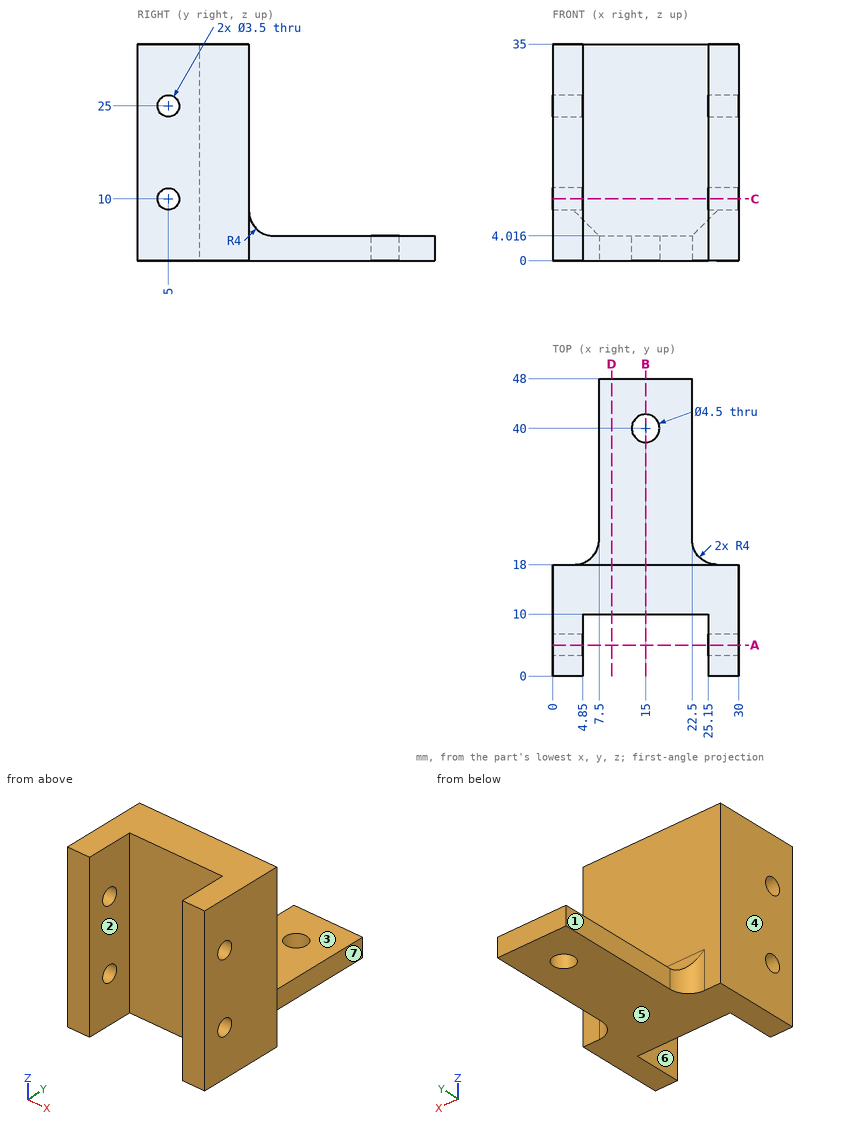
Input: dimensioned drawing with shaded views. Units: mm. Origin: part minimum x, y, z. A direction names the side the tool comes from. Round coordinates to 2 decimals unless told otherwise and drop trailing zeros. Order: outer loops, then holes, each group sorted by start corner. A loop starts at its lowest first (then second) coordinate and runs counter-clockwise, first axis right, second up.
Q1. Mould query, pull axis X, two halves, no side actions, for the marked faces 4, 5, 6 and 7. Classes: released by +X, released by -X, zero draft, split by the parting line, or undercut.
Result sheet:
face 4: released by -X
face 5: zero draft
face 6: undercut
face 7: released by +X
Q2. Section A-A, the plane y = 5. Output: boundary loops of the cut face in (x, z), and give its area (3 significant figures).
Result sheet:
outline: (0, 0) - (4.85, 0) - (4.85, 8.25) - (0, 8.25) - close; (0, 11.75) - (4.85, 11.75) - (4.85, 23.25) - (0, 23.25) - close; (0, 26.75) - (4.85, 26.75) - (4.85, 35) - (0, 35) - close; (25.15, 0) - (30, 0) - (30, 8.25) - (25.15, 8.25) - close; (25.15, 11.75) - (30, 11.75) - (30, 23.25) - (25.15, 23.25) - close; (25.15, 26.75) - (30, 26.75) - (30, 35) - (25.15, 35) - close
area: 272 mm2
Q3. Access query for the marked faces 1, 2 and 3. Directions: +Z, -Z, +X, -X, +Y, -Y. A direction counts if a zero-diameter tool reaches every point of the face in a straight line with its end or side. Return the directions, or none.
Result sheet:
face 1: +Z, -Z, -X, +Y
face 2: +Z, -Z, -Y
face 3: +Z, +X, -X, +Y
Q4. Material intervals for probe 1 along Z at (x, y) = (3.65, 5); probe 2 along Y at (x, z) = (1.25, 10); probe 3 along Y at (x, z) = (23.75, 34), sorted ascending.
Result sheet:
probe 1: z = 0 to 8.25, 11.75 to 23.25, 26.75 to 35
probe 2: y = 0 to 3.25, 6.75 to 18
probe 3: y = 10 to 18
Q5. Section C-C, the plane z = 10. Output: boundary loops of the cut face in (x, y), and give its area (3 significant figures).
Result sheet:
outline: (0, 0) - (4.85, 0) - (4.85, 3.25) - (0, 3.25) - close; (0, 6.75) - (4.85, 6.75) - (4.85, 10) - (25.15, 10) - (25.15, 6.75) - (30, 6.75) - (30, 18) - (0, 18) - close; (25.15, 0) - (30, 0) - (30, 3.25) - (25.15, 3.25) - close
area: 303 mm2
Q6. Section D-D, the plane x = 9.5. Output: boundary loops of the cut face in (y, z).
Result sheet:
outline: (10, 0) - (48, 0) - (48, 4.02) - (22, 4.02) arc R4 cw to (18, 8.02) - (18, 35) - (10, 35) - close
Q7. Section B-B, the plane x = 15. Output: boundary loops of the cut face in (y, z), and give its area (3 significant figures).
Result sheet:
outline: (10, 0) - (37.75, 0) - (37.75, 4.02) - (22, 4.02) arc R4 cw to (18, 8.02) - (18, 35) - (10, 35) - close; (42.25, 0) - (48, 0) - (48, 4.02) - (42.25, 4.02) - close
area: 386 mm2
Q8. Pin query (flat end, axial travel): pin 1 (4 mm diameter, centred on x = 7.5, y = 37.5, fed in from +Z); pin 2 (2 mm diameter, centred on y = 32.5, z = 1.5, fed in from -X); pin 3 (3 mm diameter, centred on y = 5, z = 10, fed in from +X); pin 4 (10 mm diameter, centred on x = 15.5, y = 24.5, fed in from +Z). Return the tip coordinate at first contact, or that it passes through.
Result sheet:
pin 1: stops at z = 4.02
pin 2: stops at x = 7.5
pin 3: passes through
pin 4: stops at z = 4.89
